```python
from build123d import *

# Parameters (mm, degrees)
SKETCH1_R           = 57.15
BOSS_EXTRUDE1_DEPTH = 3.175
SKETCH2_R           = 50.8
BOSS_EXTRUDE2_DEPTH = 70
SHELL3_T            = -3.81
BOSS_EXTRUDE3_REACH = 111.027
SKETCH3_W           = 39.7
SKETCH3_H           = 39.7
SKETCH3_W_2         = 27
SKETCH3_H_2         = 27
FILLET2_R           = 2.54
SKETCH4_W           = 27
SKETCH4_H           = 27
BOSS_EXTRUDE5_DEPTH = 40


with BuildPart() as part:
    # Sketch1 → Boss-Extrude1 (new body)
    with BuildSketch(Plane(origin=(0, 0, 0), x_dir=(1, 0, 0), z_dir=(0, 1, 0))):
        with Locations(Location((0, 0, 0), (0, 0, 270))):
            Circle(SKETCH1_R)
    extrude(amount=BOSS_EXTRUDE1_DEPTH)

    # Sketch2 → Boss-Extrude2 (add)
    with BuildSketch(Plane(origin=(0, 3.175, 0), x_dir=(1, 0, 0), z_dir=(0, 1, 0))):
        with Locations(Location((0, 0, 0), (0, 0, 270))):
            Circle(SKETCH2_R)
    extrude(amount=BOSS_EXTRUDE2_DEPTH)

    # Shell3
    shell3_openings = [part.faces().sort_by_distance(p)[0] for p in [
        (0, 73.175, 0),
    ]]
    offset(amount=SHELL3_T, openings=shell3_openings, kind=Kind.INTERSECTION)

    # Sketch3 → Boss-Extrude3 (add, up to next)
    with BuildSketch(Plane(origin=(0, 73.175, 0), x_dir=(1, 0, 0), z_dir=(0, 1, 0)), mode=Mode.PRIVATE) as boss_extrude3_sk1:
        Rectangle(SKETCH3_W, SKETCH3_H)
        Rectangle(SKETCH3_W_2, SKETCH3_H_2, mode=Mode.SUBTRACT)
    boss_extrude3_tool1 = extrude(boss_extrude3_sk1.sketch, amount=-BOSS_EXTRUDE3_REACH, mode=Mode.PRIVATE) - part.part
    add(boss_extrude3_tool1.solids().sort_by_distance((0, 73.175, -19.288557))[0])

    # Fillet2
    fillet2_edges = [part.edges().sort_by_distance(p)[0] for p in [
        (0, 3.175, -50.8),
        (0, 73.175, -50.8),
    ]]
    fillet(fillet2_edges, radius=FILLET2_R)

    # Sketch4 → Boss-Extrude5 (add)
    with BuildSketch(Plane(origin=(0, 3.81, 0), x_dir=(1, 0, 0), z_dir=(0, 1, 0))):
        Rectangle(SKETCH4_W, SKETCH4_H)
    extrude(amount=BOSS_EXTRUDE5_DEPTH)


solid = part.part
```
Design review of the part built by this model. Coordinates are the model's own, in mm. A direction names the side the tool comes from. Coordinates: 2 decimals unless noted, no trailing zeros. Loops run counter-clockwise (first coordinate to the right, second up) from the corner with the lowest first, then second, coordinate; pieces in that order, holes last.
Q1. For pin 1 (3 mm diameter, centred on x = -7.5, y = 21, fed in from +Z); pin 2 (13.5 mm diameter, centred on x = 4.5, y = 59, fed in from +Z); pin 3 (20 mm diameter, centred on y = 36.5, z = 1, fed in from +X), all flat-tipped, find the tip position at first contact; note any pin that passes through.
Reported:
pin 1: stops at z = 50.44
pin 2: stops at z = 50.8
pin 3: stops at x = 50.8
Q2. We need section A-A on y = 50.5. State the section outline as (x, z) points.
Reported:
outline: circle Ø101.6 at (0, 0); (-19.85, -19.85) - (19.85, -19.85) - (19.85, 19.85) - (-19.85, 19.85) - close; hole circle Ø93.98 at (0, 0); hole (-13.5, -13.5) - (13.5, -13.5) - (13.5, 13.5) - (-13.5, 13.5) - close
Q3. We need section D-D on z = 0. State the section outline as (x, y) points (3 decimals), and give its area (3 significant figures).
Reported:
outline: (-57.15, 0) - (57.15, 0) - (57.15, 3.175) - (53.34, 3.175) arc R2.54 cw to (50.8, 5.715) - (50.8, 70.635) arc R2.54 ccw to (48.26, 73.175) - (46.99, 73.175) - (46.99, 3.81) - (19.85, 3.81) - (19.85, 73.175) - (13.5, 73.175) - (13.5, 43.81) - (-13.5, 43.81) - (-13.5, 73.175) - (-19.85, 73.175) - (-19.85, 3.81) - (-46.99, 3.81) - (-46.99, 73.175) - (-48.26, 73.175) arc R2.54 ccw to (-50.8, 70.635) - (-50.8, 5.715) arc R2.54 cw to (-53.34, 3.175) - (-57.15, 3.175) - close
area: 2,920 mm2
Q4. Tool access review of faces 1 (the face through (0, 59, -13.5)), 2 (the face through (-46.2, 73.175, 10.5)): name each direction out of +Z, -Z, +X, -X, +Y, -Y from which nothing blocks a thin tool from reaching the whole face with its end or side.
Reported:
face 1: +Y
face 2: +Z, -Z, +X, -X, +Y
Q5. The part is to be moulded in two halves that separate along X. For faces 3 (the face through (2.513, 1.565, -57.095)), 4 (the face through (0, 73.175, -14)), 5 (the face through (19.85, 39, 0)), say which applies: +X half, -X half, draft (parallel to the pull), parting line (faces both ways), or undercut.
Reported:
face 3: parting line
face 4: draft
face 5: undercut
Q6. We need section C-C on x = 0. State the section outline as (y, z) points (3 decimals).
Reported:
outline: (0, -57.15) - (3.175, -57.15) - (3.175, -53.34) arc R2.54 cw to (5.715, -50.8) - (70.635, -50.8) arc R2.54 ccw to (73.175, -48.26) - (73.175, -46.99) - (3.81, -46.99) - (3.81, -19.85) - (73.175, -19.85) - (73.175, -13.5) - (43.81, -13.5) - (43.81, 13.5) - (73.175, 13.5) - (73.175, 19.85) - (3.81, 19.85) - (3.81, 46.99) - (73.175, 46.99) - (73.175, 48.26) arc R2.54 ccw to (70.635, 50.8) - (5.715, 50.8) arc R2.54 cw to (3.175, 53.34) - (3.175, 57.15) - (0, 57.15) - close
Q7. To check wall thickness, follow line 1 (X direction, y = 51, z = 0); line 2 (X direction, y = 25, z = 0); line 3 (X direction, y = 44, z = 3). State the ranges of each line that lie inside material, in increasing order.
Reported:
line 1: x = -50.8 to -46.99, -19.85 to -13.5, 13.5 to 19.85, 46.99 to 50.8
line 2: x = -50.8 to -46.99, -19.85 to 19.85, 46.99 to 50.8
line 3: x = -50.71 to -46.89, -19.85 to -13.5, 13.5 to 19.85, 46.89 to 50.71
Q8. We need section B-B on y = 27.5. State the section outline as (x, z) points.
Reported:
outline: circle Ø101.6 at (0, 0); (-19.85, -19.85) - (19.85, -19.85) - (19.85, 19.85) - (-19.85, 19.85) - close; hole circle Ø93.98 at (0, 0)
